Geometry check sheet. Reference: the model listing, model coordinates, mm. Round coordinates to 2 decimals unless told otherwise and drop trailing zeros. Write each loop counter-clockwise with the first axis right and the second up, starting at its lowest first coordinate (ties: lowest second). Pieces come first, ordered by that corner, then holes.
Item 1: Cross-section at C-C (x = 10.75). Enter the section's corners in (y, z), then the cut area to 3 significant figures.
Item 2: Draft check along Y on faces 1 (the face through (10.65, 3.27, -10.4)), 2 (the face through (10.86, -14.334, -9.139)), 3 (the face through (1, -9, -15)). Enter one of: pulls with the +Y half, pulls with the -Y half, needs draft (parallel to the pull), parting line crosses it, or undercut.
Item 3: Depth check by flat-ended pin: P1, Ø4, axis at x = 11, z = 11, coming from the +Y side; P2, Ø2, axis at x = 8, z = -15, coming from the +Y side; P3, Ø1.5, axis at x = 7, z = -8, coming from the -Y side. Enter the tip coordinate at first touch or a pass-through.
Item 4: Cross-section at D-D (y = 17.5). Enter the section's corners in (x, z).
Item 5: Cross-section at A-A (z = 0). Enter the section's corners in (x, y).
Item 6: Scan lines: probe 1 along Y at (x, z) = (11, 0); probe 2 along X at (y, z) = (-17, -6.5); probe 3 along Y at (x, z) = (3.25, 1.5). Record each from-to range of solid material in increasing order.
Autodesk Inventor part; units mm, degrees
ref_plane "YZ Plane" through (0, 0, 0) normal (1, 0, 0) x (0, 1, 0)
ref_plane "XZ Plane" through (0, 0, 0) normal (0, 1, 0) x (-1, 0, 0)
ref_plane "XY Plane" through (0, 0, 0) normal (0, 0, 1) x (1, 0, 0)
sketch "Skizze1" plane through (0, 0, 0) normal (1, 0, 0) x (0, 1, 0)
  circle A0 centre (0, 0) radius 20
  dimension "d0" = 40
extrude "Extrusion1" add sketch "Skizze1" along normal blind 1
sketch "Skizze2" plane through (1, 0, 0) normal (1, 0, 0) x (0, 0, -1)
  circle A0 centre (0, 0) radius 20
  circle A1 centre (0, 0) radius 17
  dimension "d3" = 34
extrude "Extrusion2" add sketch "Skizze2" along normal blind 20 contours A1
sketch "Skizze5" plane through (0, 0, 0) normal (-1, 0, 0) x (0, 0, 1)
  circle A0 centre (0, 0) radius 20
  circle A1 centre (0, 0) radius 5
  dimension "d12" = 10
extrude "Extrusion5" add sketch "Skizze5" along normal blind 10 contours A1
sketch "Skizze6" plane through (21, 0, 0) normal (1, 0, 0) x (0, 0, -1)
  circle A0 centre (0, 0) radius 17
  circle A1 centre (0, 0) radius 10.9
  dimension "d15" = 21.8
extrude "Extrusion6" cut sketch "Skizze6" against normal through all contours A1
properties part number "Rolle_schieber21.8 ipt"
Resolved:
1. outline: circle Ø34 at (0, 0); hole circle Ø21.8 at (0, 0)
1. area: 535 mm2
2. face 1: undercut
2. face 2: parting line crosses it
2. face 3: needs draft
3. P1: stops at y = 14.42
3. P2: stops at y = 9.64
3. P3: stops at y = -15.38
4. outline: (0, -9.68) - (1, -9.68) - (1, 9.68) - (0, 9.68) - close
5. outline: (0, -20) - (1, -20) - (1, -17) - (21, -17) - (21, -10.9) - (0, -10.9) - close; (0, 10.9) - (21, 10.9) - (21, 17) - (1, 17) - (1, 20) - (0, 20) - close
6. probe 1: y = -17 to -10.9, 10.9 to 17
6. probe 2: x = 0 to 1
6. probe 3: y = -16.93 to -10.8, 10.8 to 16.93
